Source: CAD feature listing. Evaluate the final solid. Frame: model axes, mm. Round coordinates to 2 decimals unless told otherwise and drop trailing zeros. Order: outer loops, then holes, each group sorted by start corner. A loop starts at its lowest first (then second) coordinate and runs counter-clockwise, first axis right, second up. Notation, with made-up numbers: (76, 69) -> (104, 69) arc R6 ccw to (104, 75) -> close; hole circle Ø2 at (46.5, -31). An arc over 180 degrees is marked (long way). Use a Markdown table: item, result. Add a question column.
```python
from build123d import *

# Parameters (mm, degrees)
BOSS_EXTRUDE1_DEPTH  = 3.175
SKETCH4_R            = 4
LEFT_AND_RIGHT_DEPTH = 363.060140032


with BuildPart() as part:
    # Sketch1 → Boss-Extrude1 (new, symmetric)
    with BuildSketch(Plane(origin=(0, 0, 0), x_dir=(1, 0, 0), z_dir=(0, 1, 0))):
        Polygon((-354.15, 75), (-354.15, -75), (-260.5, -75), (-260.5, -68.65), (260.5, -68.65), (260.5, -75), (354.15, -75), (354.15, 75), (260.5, 75), (260.5, 68.65), (-260.5, 68.65), (-260.5, 75), align=None)
    extrude(amount=BOSS_EXTRUDE1_DEPTH, both=True)

    # Sketch4 → Left and Right (cut, through all)
    with BuildSketch(Plane.XZ.offset(3.175)):
        with Locations(Location((-326.1, 14.85, 0), (0, 0, 270))):
            Circle(SKETCH4_R)
        with Locations(Location((205.9, 14.85, 0), (0, 0, 270))):
            Circle(SKETCH4_R)
    extrude(amount=-LEFT_AND_RIGHT_DEPTH, mode=Mode.SUBTRACT)


solid = part.part
```
1) First-contact query: pin 1 Ø1.9 at (x, y) = (84, 1) entering from -Z. Flat tip, straight axial feed; report the tip coordinate or a pass-through.
2) Line query: probe 1 along X at (y, z) = (-0.75, 14.85); probe 2 along Z at (x, y) = (-326.1, -0.25); probe 3 along Z at (x, y) = (58, 3). Output: solid intervals per line, ascending. Write a range as from..to.
3) Section A-A on y = 0.5. Output: boundary loops of the cut face in (x, z).
4) Draft query along Y for faces 1 (the flat face through (-5, 3.175, -1)), 2 (the flat face through (-5, -3.175, -1)). Return one class per face: pulls with the +Y half, pulls with the -Y half, needs draft (parallel to the pull), parting line crosses it, or undercut.
5) Section B-B on x = 226. Output: boundary loops of the cut face in (y, z) (3 decimals), then the cut area to 3 significant figures.
Conclusion:
| question | item | result |
|---|---|---|
| 1 | pin 1 | stops at z = -68.65 |
| 2 | probe 1 | x = -354.15..-330.1, -322.1..201.9, 209.9..354.15 |
| 2 | probe 2 | z = -75..10.85, 18.85..75 |
| 2 | probe 3 | z = -68.65..68.65 |
| 3 | outline | (-354.15, -75) -> (-260.5, -75) -> (-260.5, -68.65) -> (260.5, -68.65) -> (260.5, -75) -> (354.15, -75) -> (354.15, 75) -> (260.5, 75) -> (260.5, 68.65) -> (-260.5, 68.65) -> (-260.5, 75) -> (-354.15, 75) -> close; hole circle Ø8 at (-326.1, 14.85); hole circle Ø8 at (205.9, 14.85) |
| 4 | face 1 | pulls with the +Y half |
| 4 | face 2 | pulls with the -Y half |
| 5 | outline | (-3.175, -68.65) -> (3.175, -68.65) -> (3.175, 68.65) -> (-3.175, 68.65) -> close |
| 5 | area | 872 mm^2 |
